For this review, take the finished solid that the model builds, in its own axes (mm). Give positions to 0.01 mm unless a question says otherwise; leave off trailing zeros. Order: outer loops, then holes, each group sorted by start corner. A loop starts at its lowest first (then second) coordinate and runs counter-clockwise, first axis right, second up. Notation, with made-up numbers: (74, 70.25) - (125, 70.25) arc R30 cw to (125, 95.25) - close; hole circle Ø4 at (46.5, -12). An arc over 180 degrees is marked (long way). One line per item, written item: value.
```python
from build123d import *

# Parameters (mm, degrees)
SKETCH_1_R               = 80
EXTRUDE_1_DEPTH          = 5
CUT_EXTRUDE_3_DEPTH      = 114.247516529
PATTERN_CIRCULAR_2_COUNT = 6
SKETCH_2_R               = 7
SKETCH_2_R_2             = 2
EXTRUDE_2_DEPTH          = 10


with BuildPart() as part:
    # Sketch 1 → Extrude 1 (new body)
    with BuildSketch(Plane(origin=(0, 0, 0), x_dir=(1, 0, 0), z_dir=(0, 1, 0))):
        with Locations(Location((0, 0, 0), (0, 0, 270))):
            Circle(SKETCH_1_R)
    extrude(amount=EXTRUDE_1_DEPTH)

    # Sketch 5 → Cut-Extrude 3 (cut, through all)
    with BuildSketch(Plane(origin=(0, 5, 0), x_dir=(1, 0, 0), z_dir=(0, 1, 0))):
        with BuildLine():
            Line((-41.607553791, 17.140929599), (-11.557653831, 4.761369333))
            ThreePointArc((-11.557653831, 4.761369333), (-9.232157797, 8.427174047), (-5.79312728, 11.076537199))
            Line((-5.79312728, 11.076537199), (-20.855258209, 39.875533916))
            ThreePointArc((-20.855258209, 39.875533916), (-33.235768068, 30.337826569), (-41.607553791, 17.140929599))
        make_face()
    cut_extrude_3 = extrude(amount=-CUT_EXTRUDE_3_DEPTH, mode=Mode.SUBTRACT)

    # Pattern Circular 2: Cut-Extrude 3 ×6 about axis
    pattern_circular_2_axis = Axis((0, 0, 0), (0, 1, 0))
    for i in range(1, PATTERN_CIRCULAR_2_COUNT):
        add(cut_extrude_3.rotate(pattern_circular_2_axis, i * 360 / PATTERN_CIRCULAR_2_COUNT), mode=Mode.SUBTRACT)

    # Sketch 2 → Extrude 2 (add)
    with BuildSketch(Plane(origin=(0, 5, 0), x_dir=(1, 0, 0), z_dir=(0, 1, 0))):
        with Locations(Location((0, 0, 0), (0, 0, 270))):
            Circle(SKETCH_2_R)
        with Locations(Location((0, 0, 0), (0, 0, 270))):
            Circle(SKETCH_2_R_2, mode=Mode.SUBTRACT)
    extrude(amount=EXTRUDE_2_DEPTH)


solid = part.part
```
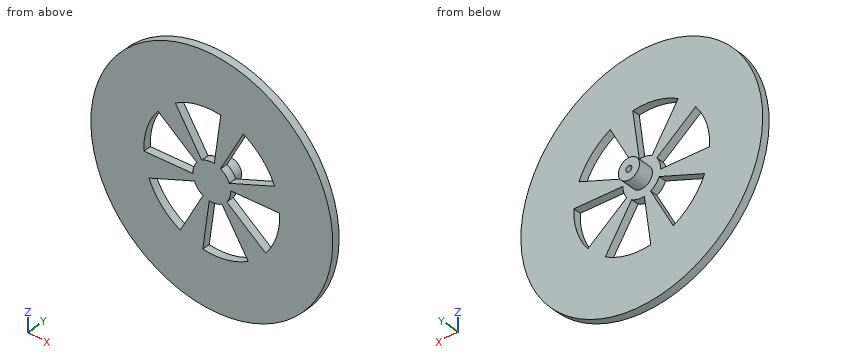
(1) Take a section at A-A (z = -35.5). Write out the cut boundary in (x, y).
Answers below:
outline: (-71.69, 0) - (-27.65, 0) - (-27.65, 5) - (-71.69, 5) - close; (-18.57, 0) - (-4.74, 0) - (-4.74, 5) - (-18.57, 5) - close; (22.52, 0) - (71.69, 0) - (71.69, 5) - (22.52, 5) - close
(2) Take a section at C-C (x = 16.5). Write out the cut boundary in (y, z).
Answers below:
outline: (0, -78.28) - (5, -78.28) - (5, -41.87) - (0, -41.87) - close; (0, -26.01) - (5, -26.01) - (5, -12.71) - (0, -12.71) - close; (0, 0.69) - (5, 0.69) - (5, 6.8) - (0, 6.8) - close; (0, 31.55) - (5, 31.55) - (5, 78.28) - (0, 78.28) - close
(3) Wall thickness on line 1 (X direction, y = 11, z = 0); line 2 (Z direction, x = 9.5, y = 0.5); line 3 (Y direction, x = -1, z = 47.5): over which ranges is each line inside the solid? List them lowest first. Write a range as from..to.
Answers below:
line 1: x = -7..-2, 2..7
line 2: z = -79.43..-43.99, -14.98..8.12, 18.16..79.43
line 3: y = 0..5
(4) Take a section at B-B (y = 3). Write out the cut boundary in (x, z), then the cut area to 3 significant figures.
Answers below:
outline: circle Ø160 at (0, 0); hole (-44.96, -1.88) - (-12.49, -0.52) arc R12.5 cw to (-9.9, 7.63) - (-35.65, 27.46) arc R45 ccw to start; hole (-41.61, -17.14) arc R45 ccw to (-20.86, -39.88) - (-5.79, -11.08) arc R12.5 cw to (-11.56, -4.76) - close; hole (-24.11, 38) - (-6.7, 10.56) arc R12.5 cw to (1.66, 12.39) - (5.96, 44.6) arc R45 ccw to start; hole (-5.96, -44.6) arc R45 ccw to (24.11, -38) - (6.7, -10.56) arc R12.5 cw to (-1.66, -12.39) - close; hole (5.79, 11.08) arc R12.5 cw to (11.56, 4.76) - (41.61, 17.14) arc R45 ccw to (20.86, 39.88) - close; hole (9.9, -7.63) - (35.65, -27.46) arc R45 ccw to (44.96, 1.88) - (12.49, 0.52) arc R12.5 cw to start
area: 16,200 mm^2
(5) Take a section at D-D (z = 20.5). Write out the cut boundary in (x, y), then the cut area to 3 significant figures.
Answers below:
outline: (-77.33, 0) - (-40.06, 0) - (-40.06, 5) - (-77.33, 5) - close; (-26.61, 0) - (-13, 0) - (-13, 5) - (-26.61, 5) - close; (2.74, 0) - (10.72, 0) - (10.72, 5) - (2.74, 5) - close; (40.06, 0) - (77.33, 0) - (77.33, 5) - (40.06, 5) - close
area: 481 mm^2
(6) For P1, Ø8, axis at y = 1.5, z = -24, coming from the -X side; P2, Ø2, axis at x = 44.5, y = 4.5, coming from the -Z side; P3, Ø5, axis at y = 6.5, z = -39, coming from the -X side, all flat-tipped, find the tip position at first contact; note any pin that passes through.
Answers below:
P1: stops at x = -77.46
P2: stops at z = -67.14
P3: stops at x = -70.93
